Could you check a few things on this model? Use its own coordinates, in mm. Coordinates: 2 decimals unless noted, no trailing zeros. Write each loop counter-clockwise with the first axis right and the second up, starting at its lowest first coordinate (ties: lowest second). Pieces come first, ordered by that corner, then holes.
Item 1: For P1, Ø3, axis at x = -8.5, z = 12.5, coming from the -Y side; P2, Ø4, axis at y = -3, z = -4, coming from the -X side; P3, Ø4, axis at x = 3.5, y = -2, coming from the +Z side; P4, Ø12, axis at x = -6, y = 4.5, coming from the -Z side, each with a flat end and sliding along its axis, tell me the tip position at first contact or that it passes through.
Item 2: I want a section at A-A on z = 21. Please give me the cut outline in (x, y), then the cut area to 3 significant figures.
Item 3: If I drill on probe 1 along Y at (x, z) = (-0.5, -17.5); probe 2 along Y at (x, z) = (-4.25, -12.5); probe 3 along X at (y, z) = (1.25, -74), over which ranges is the centre line in solid material (lowest first)?
from build123d import *

# Parameters (mm, degrees)
F0_R       = 12.7
F1_DEPTH   = 63.5
F2_R       = 12.7
F6_R       = 120.1325893594
F1_FACE1_R = 12.7
F8_R       = 9.525
F10_R      = 3.81


with BuildPart() as f1:
    # F0 (on Top) → F1 (new body, symmetric)
    with BuildSketch(Plane.XY):
        Circle(F0_R)
    extrude(amount=F1_DEPTH, both=True)

    # F2 (on face) → F5 section 0
    with BuildSketch(Plane.XY.offset(63.5), mode=Mode.PRIVATE) as f5_s0:
        Circle(F2_R)
    loft([Vertex(0, 0, 88.9), f5_s0.sketch])

    # F6
    f6_edges = [f1.edges().sort_by_distance(p)[0] for p in [
        (6.35, 0, 76.2),
        (-12.7, 0, 63.5),
    ]]
    fillet(f6_edges, radius=F6_R)

    # F1_face1 (on face) → F9 section 0
    with BuildSketch(Plane(origin=(0, 0, -63.5), x_dir=(1, 0, 0), z_dir=(0, 0, -1))):
        Circle(F1_FACE1_R)
    # F8 (on offset) → F9 section 1
    with BuildSketch(Plane(origin=(0, 0, -88.9), x_dir=(1, 0, 0), z_dir=(0, 0, -1))):
        Circle(F8_R)
    loft()

    # F10
    f10_edges = [f1.edges().sort_by_distance(p)[0] for p in [
        (-12.7, 0, -63.5),
        (11.1125, 0, -76.2),
        (-9.525, 0, -88.9),
    ]]
    fillet(f10_edges, radius=F10_R)


solid = f1.part
Response values:
1. P1: stops at y = -10.6
1. P2: stops at x = -12.66
1. P3: stops at z = 84.63
1. P4: stops at z = -88.9
2. outline: circle Ø25.4 at (0, 0)
2. area: 507 mm2
3. probe 1: y = -12.69 to 12.69
3. probe 2: y = -11.97 to 11.97
3. probe 3: x = -11.32 to 11.32
